Geometry check sheet. Reference: the model listing, model coordinates, mm. Coordinates: 2 decimals unless noted, no trailing zeros. Write each loop counter-clockwise with the first axis right and the second up, starting at its lowest first coordinate (ties: lowest second). Pieces come first, ordered by that corner, then holes. Notation, with made-up numbers: M 16.5,33 L 28.5,33 A22 cw 28.5,50 Z; hole C 63.5,21 d2. An arc over 180 degrees is marked long. Put each result on its own line as item: value. Start each with the question number.
1) Cross-section at A-A on z = 1. Record the cut outline in (x, y) (3 decimals), plus the area to 3 significant figures.
2) Scan lines: line 1 along X through (y, z) = (7.5, 1.8); line 2 along X through (y, z) = (15, 1.15); line 3 along Y through (x, z) = (23, 1.4). Record each from-to range of solid material in increasing order.
3) Cross-section at C-C on x = -7.5. Record the cut outline in (y, z) (3 decimals), plus the area to 3 significant figures.
4) Gauge pin test, flat ends, axial feed: pin 1 (4 mm diameter, centred on x = 8, y = -8, fed in from -Z); pin 2 (0.8 mm diameter, centred on y = 10, z = 2, fed in from +X); pin 3 (1.4 mm diameter, centred on y = -13, z = 0.5, fed in from -X); pin 4 (1.5 mm diameter, centred on x = 27.5, z = 0.5, fed in from -Y). Record the tip position at first contact, or that the pin passes through.
5) Cross-section at D-D on x = 29. Record the cut outline in (y, z), plus the area to 3 significant figures.
6) Cross-section at B-B on y = 4. Record the cut outline in (x, z), plus the area to 3 significant figures.
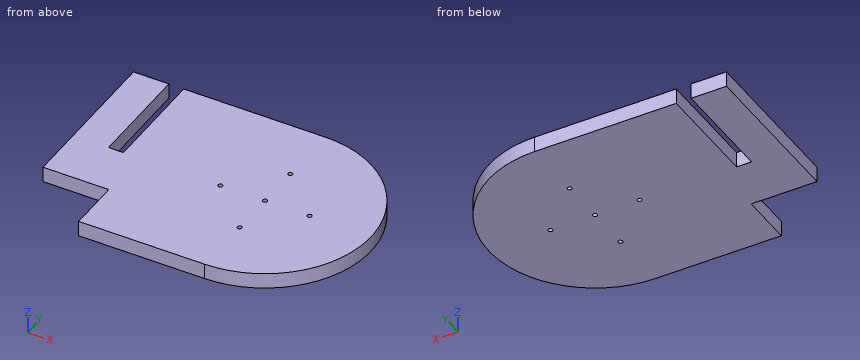
from build123d import *

# Parameters (mm, degrees)
SKETCH1_R           = 0.396875
BOSS_EXTRUDE1_DEPTH = 2.794


with BuildPart() as part:
    # Sketch1 → Boss-Extrude1 (new body)
    with BuildSketch(Plane.XY):
        with BuildLine():
            Line((-6.728072382, 19.05), (18.671927618, 19.05))
            ThreePointArc((18.671927618, 19.05), (37.721927618, 0), (18.671927618, -19.05))
            Line((18.671927618, -19.05), (-3.934072382, -19.05))
            Line((-3.934072382, -19.05), (-3.934072382, -9.525))
            Line((-3.934072382, -9.525), (-15.745072382, -9.525))
            Line((-15.745072382, -9.525), (-15.745072382, 19.05))
            Line((-15.745072382, 19.05), (-9.395072382, 19.05))
            Line((-9.395072382, 19.05), (-9.395072382, 0))
            Line((-9.395072382, 0), (-6.728072382, 0))
            Line((-6.728072382, 0), (-6.728072382, 19.05))
        make_face()
        with Locations((18.671927618, 8)):
            Circle(SKETCH1_R, mode=Mode.SUBTRACT)
        with Locations((18.671927618, 0)):
            Circle(SKETCH1_R, mode=Mode.SUBTRACT)
        with Locations((26.671927618, 0)):
            Circle(SKETCH1_R, mode=Mode.SUBTRACT)
        with Locations((18.671927618, -8)):
            Circle(SKETCH1_R, mode=Mode.SUBTRACT)
        with Locations((10.671927618, 0)):
            Circle(SKETCH1_R, mode=Mode.SUBTRACT)
    extrude(amount=BOSS_EXTRUDE1_DEPTH)


solid = part.part
Answer key:
1. outline: M -15.745,-9.525 L -3.934,-9.525 L -3.934,-19.05 L 18.672,-19.05 A19.05 ccw 18.672,19.05 L -6.728,19.05 L -6.728,0 L -9.395,0 L -9.395,19.05 L -15.745,19.05 Z; hole C 10.672,0 d0.794; hole C 18.672,-8 d0.794; hole C 18.672,0 d0.794; hole C 18.672,8 d0.794; hole C 26.672,0 d0.794
1. area: 1,720 mm²
2. line 1: x = -15.75 to -9.4, -6.73 to 36.18
2. line 2: x = -15.75 to -9.4, -6.73 to 30.42
2. line 3: y = -18.55 to 18.55
3. outline: M -9.525,0 L 0,0 L 0,2.794 L -9.525,2.794 Z
3. area: 26.6 mm²
4. pin 1: stops at z = 0
4. pin 2: stops at x = 35.13
4. pin 3: stops at x = -3.93
4. pin 4: stops at y = -17.25
5. outline: M -16.01,0 L 16.01,0 L 16.01,2.79 L -16.01,2.79 Z
5. area: 89.4 mm²
6. outline: M -15.75,0 L -9.4,0 L -9.4,2.79 L -15.75,2.79 Z; M -6.73,0 L 37.3,0 L 37.3,2.79 L -6.73,2.79 Z
6. area: 141 mm²
